Build history of the part. All positions in model axes, mm. Round coordinates to 2 decimals unless told otherwise and drop trailing zeros. Write each loop counter-clockwise with the first axis right and the second up, starting at its lowest first coordinate (ties: lowest second). Pieces come first, ordered by that corner, then holes. Notation, with made-up numbers: (33.5, 74) -> (84.5, 74) arc R31 ccw to (84.5, 103) -> close; hole circle Ø7 at (80, 1). An arc over 180 degrees is marked (long way). Answer in a Markdown table with one row per item.
```python
from build123d import *

# Parameters (mm, degrees)
SKETCH_1_W          = 58.128760995
SKETCH_1_H          = 85
SKETCH_1_R          = 3.175
EXTRUDE_1_DEPTH     = 3.5
SKETCH_2_R          = 2
CUT_EXTRUDE_1_DEPTH = 53.503533215


with BuildPart() as part:
    # Эскиз1 → Вытянуть1 (new body)
    with BuildSketch(Plane(origin=(0, 0, 0), x_dir=(1, 0, 0), z_dir=(0, 1, 0))):
        with Locations((-1.564380498, 0)):
            Rectangle(SKETCH_1_W, SKETCH_1_H)
        with Locations(Location((0, 0, 0), (0, 0, 270))):
            Circle(SKETCH_1_R, mode=Mode.SUBTRACT)
    extrude(amount=EXTRUDE_1_DEPTH)

    # Эскиз2 → Вырез-Вытянуть1 (cut, through all)
    with BuildSketch(Plane(origin=(0, 3.5, 0), x_dir=(1, 0, 0), z_dir=(0, 1, 0))):
        with Locations(Location((-5.945819696, 2.881931911, 0), (0, 0, 270))):
            Circle(SKETCH_2_R)
        with Locations(Location((5.945819696, -2.881931911, 0), (0, 0, 270))):
            Circle(SKETCH_2_R)
        with Locations(Location((20.247006678, -9.813700656, 0), (0, 0, 270))):
            Circle(SKETCH_2_R)
        with Locations(Location((9.813700656, 20.247006678, 0), (0, 0, 270))):
            Circle(SKETCH_2_R)
        with Locations(Location((-9.813700656, -20.247006678, 0), (0, 0, 270))):
            Circle(SKETCH_2_R)
        with Locations(Location((-20.247006678, 9.813700656, 0), (0, 0, 270))):
            Circle(SKETCH_2_R)
    extrude(amount=-CUT_EXTRUDE_1_DEPTH, mode=Mode.SUBTRACT)


solid = part.part
```
Q1. Wall check: line 1 (X direction, y = 2.3, z = 0) (3 decimals); line 2 (X direction, y = 0.7, z = -2.5); line 3 (Z direction, x = -9, y = 2.5). Give the ranges that are in metal, low to high. Write a range as [from, to].
A:
| item | result |
|---|---|
| line 1 | [-30.629, -3.175], [3.175, 27.5] |
| line 2 | [-30.63, -7.91], [-3.98, -1.96], [1.96, 27.5] |
| line 3 | [-42.5, 18.42], [22.07, 42.5] |
Q2. Saw through at C-C on y = 1.4. Write the cut outline in (x, z) (3 decimals), plus the area to 3 significant figures.
A:
| item | result |
|---|---|
| outline | (-30.629, -42.5) -> (27.5, -42.5) -> (27.5, 42.5) -> (-30.629, 42.5) -> close; hole circle Ø4 at (-20.247, -9.814); hole circle Ø4 at (-9.814, 20.247); hole circle Ø4 at (-5.946, -2.882); hole circle Ø6.35 at (0, 0); hole circle Ø4 at (5.946, 2.882); hole circle Ø4 at (9.814, -20.247); hole circle Ø4 at (20.247, 9.814) |
| area | 4,830 mm² |
Q3. Drop a flat-ended pin along its axis: P1, Ø10, axis at x = -13.5, z = 28, coming from the -Y side. Give the stop position or say it passes through.
A:
| item | result |
|---|---|
| P1 | y = 0 |
Q4. Two-plate mould, pull along Z, no slides. Class faces 1 (the flat face through (4, 0, -1)), 2 (the flat face through (-2, 2, -42.5)), 3 (the cylindrical face through (-11.03, 1.77, 18.66)): released by +Z, released by -Z, zero draft, split by the parting line, or undercut.
A:
| item | result |
|---|---|
| face 1 | zero draft |
| face 2 | released by -Z |
| face 3 | undercut |
Q5. Saw through at B-B on z = 0. Write the cut outline in (x, y) (3 decimals), plus the area to 3 significant figures.
A:
| item | result |
|---|---|
| outline | (-30.629, 0) -> (-3.175, 0) -> (-3.175, 3.5) -> (-30.629, 3.5) -> close; (3.175, 0) -> (27.5, 0) -> (27.5, 3.5) -> (3.175, 3.5) -> close |
| area | 181 mm² |
Q6. Saw through at A-A on x = 0. Write the cut outline in (y, z) (3 decimals).
A:
| item | result |
|---|---|
| outline | (0, -42.5) -> (3.5, -42.5) -> (3.5, -3.175) -> (0, -3.175) -> close; (0, 3.175) -> (3.5, 3.175) -> (3.5, 42.5) -> (0, 42.5) -> close |
